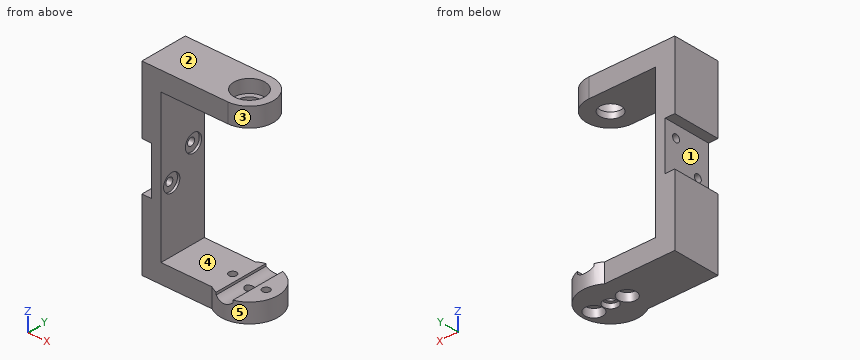
```python
from build123d import *

# Parameters (mm, degrees)
SZKIC25_W                        = 62.15
SZKIC25_H                        = 20
DODANIE_WYCI_GNI_CIE7_DEPTH      = 8
SZKIC14_R                        = 1.75
DODANIE_WYCI_GNI_CIE5_DEPTH      = 8
SZKIC16_R                        = 4.5
DODANIE_WYCI_GNI_CIE6_DEPTH      = 8
SZKIC19_R                        = 6.5
WYTNIJ_WYCI_GNI_CIE8_DEPTH       = 5.5
WYTNIJ_WYCI_GNI_CIE9_REACH       = 94.496
SZKIC20_R                        = 1.6
SZKIC21_R                        = 3.75
WYTNIJ_WYCI_GNI_CIE10_DEPTH      = 3.5
SZKIC22_R                        = 3
WYTNIJ_WYCI_GNI_CIE11_DEPTH      = 2
WYTNIJ_WYCI_GNI_CIE12_REACH      = 68.384
WYTNIJ_WYCI_GNI_CIE12_END_RADIUS = 12
SZKIC26_W                        = 20.2
SZKIC26_H                        = 20
WYTNIJ_WYCI_GNI_CIE13_DEPTH      = 4
WYTNIJ_WYCI_GNI_CIE14_REACH      = 62.057
SZKIC27_R                        = 1.6
SZKIC28_R                        = 3.75
WYTNIJ_WYCI_GNI_CIE15_DEPTH      = 1


with BuildPart() as part:
    # Szkic25 → Dodanie-wyciągnięcie7 (new body)
    with BuildSketch(Plane(origin=(0, 0, 0), x_dir=(0, 0, -1), z_dir=(1, 0, 0))):
        Rectangle(SZKIC25_W, SZKIC25_H)
    extrude(amount=DODANIE_WYCI_GNI_CIE7_DEPTH)

    # Szkic14 → Dodanie-wyciągnięcie5 (add)
    with BuildSketch(Plane(origin=(0, 0, -31.075), x_dir=(-1, 0, 0), z_dir=(0, 0, -1))):
        with BuildLine():
            Line((0, 10), (0, -10))
            Line((0, -10), (-29.366750419, -10))
            ThreePointArc((-29.366750419, -10), (-48, 0), (-29.366750419, 10))
            Line((-29.366750419, 10), (0, 10))
        make_face()
        with Locations((-36, 0)):
            Circle(SZKIC14_R, mode=Mode.SUBTRACT)
    extrude(amount=DODANIE_WYCI_GNI_CIE5_DEPTH)

    # Szkic16 → Dodanie-wyciągnięcie6 (add)
    with BuildSketch(Plane.XY.offset(31.075)):
        with BuildLine():
            Line((0, 10), (0, -10))
            Line((0, -10), (36, -10))
            ThreePointArc((36, -10), (46, 0), (36, 10))
            Line((36, 10), (0, 10))
        make_face()
        with Locations((36, 0)):
            Circle(SZKIC16_R, mode=Mode.SUBTRACT)
    extrude(amount=DODANIE_WYCI_GNI_CIE6_DEPTH)

    # Szkic19 → Wytnij-wyciągnięcie8 (cut)
    with BuildSketch(Plane.XY.offset(39.075)):
        with Locations((36, 0)):
            Circle(SZKIC19_R)
    extrude(amount=-WYTNIJ_WYCI_GNI_CIE8_DEPTH, mode=Mode.SUBTRACT)

    # Szkic20 → Wytnij-wyciągnięcie9 (cut, up to next)
    with BuildSketch(Plane(origin=(0, 0, -39.075), x_dir=(-1, 0, 0), z_dir=(0, 0, -1)), mode=Mode.PRIVATE) as wytnij_wyci_gni_cie9_sk1:
        with Locations(Location((-29, 0, 0), (0, 0, 90))):
            Circle(SZKIC20_R)
    wytnij_wyci_gni_cie9_tool1 = extrude(wytnij_wyci_gni_cie9_sk1.sketch, amount=-WYTNIJ_WYCI_GNI_CIE9_REACH, mode=Mode.PRIVATE) & part.part
    # Szkic20 → Wytnij-wyciągnięcie9 (cut, up to next)
    with BuildSketch(Plane(origin=(0, 0, -39.075), x_dir=(-1, 0, 0), z_dir=(0, 0, -1)), mode=Mode.PRIVATE) as wytnij_wyci_gni_cie9_sk2:
        with Locations(Location((-43, 0, 0), (0, 0, 90))):
            Circle(SZKIC20_R)
    wytnij_wyci_gni_cie9_tool2 = extrude(wytnij_wyci_gni_cie9_sk2.sketch, amount=-WYTNIJ_WYCI_GNI_CIE9_REACH, mode=Mode.PRIVATE) & part.part
    add(wytnij_wyci_gni_cie9_tool1.solids().sort_by_distance((29, 0, -39.075))[0], mode=Mode.SUBTRACT)
    add(wytnij_wyci_gni_cie9_tool2.solids().sort_by_distance((43, 0, -39.075))[0], mode=Mode.SUBTRACT)

    # Szkic21 → Wytnij-wyciągnięcie10 (cut)
    with BuildSketch(Plane(origin=(0, 0, -39.075), x_dir=(-1, 0, 0), z_dir=(0, 0, -1))):
        with Locations(Location((-43, 0, 0), (0, 0, 90))):
            Circle(SZKIC21_R)
        with Locations(Location((-29, 0, 0), (0, 0, 90))):
            Circle(SZKIC21_R)
    extrude(amount=-WYTNIJ_WYCI_GNI_CIE10_DEPTH, mode=Mode.SUBTRACT)

    # Szkic22 → Wytnij-wyciągnięcie11 (cut)
    with BuildSketch(Plane(origin=(0, 0, -39.075), x_dir=(-1, 0, 0), z_dir=(0, 0, -1))):
        with Locations(Location((-36, 0, 0), (0, 0, 90))):
            Circle(SZKIC22_R)
    extrude(amount=-WYTNIJ_WYCI_GNI_CIE11_DEPTH, mode=Mode.SUBTRACT)

    # Wytnij-wyciągnięcie12: up to this cylinder (the profile starts inside it)
    wytnij_wyci_gni_cie12_end = Plane(origin=(36, 0, -32.110303), z_dir=(0, 0, 1)) * Cylinder(WYTNIJ_WYCI_GNI_CIE12_END_RADIUS, 161.768, mode=Mode.PRIVATE)
    # Szkic23 → Wytnij-wyciągnięcie12 (cut, up to the surface)
    with BuildSketch(Plane(origin=(0, 12, 0), x_dir=(1, 0, 0), z_dir=(0, 1, 0)), mode=Mode.PRIVATE) as wytnij_wyci_gni_cie12_sk1:
        with BuildLine():
            Line((32.5, 31.075), (39.5, 31.075))
            Line((39.5, 31.075), (39.5, 32.075))
            ThreePointArc((39.5, 32.075), (36, 33.504285786), (32.5, 32.075))
            Line((32.5, 32.075), (32.5, 31.075))
        make_face()
    wytnij_wyci_gni_cie12_tool1 = extrude(wytnij_wyci_gni_cie12_sk1.sketch, amount=-WYTNIJ_WYCI_GNI_CIE12_REACH, mode=Mode.PRIVATE) & wytnij_wyci_gni_cie12_end
    add(wytnij_wyci_gni_cie12_tool1.solids().sort_by_distance((36, 12, -32.110303))[0], mode=Mode.SUBTRACT)

    # Szkic26 → Wytnij-wyciągnięcie13 (cut)
    with BuildSketch(Plane.ZY):
        with Locations((0.7, 0)):
            Rectangle(SZKIC26_W, SZKIC26_H)
    extrude(amount=-WYTNIJ_WYCI_GNI_CIE13_DEPTH, mode=Mode.SUBTRACT)

    # Szkic27 → Wytnij-wyciągnięcie14 (cut, up to next)
    with BuildSketch(Plane.ZY.offset(-4), mode=Mode.PRIVATE) as wytnij_wyci_gni_cie14_sk1:
        with Locations((5.7, 5)):
            Circle(SZKIC27_R)
    wytnij_wyci_gni_cie14_tool1 = extrude(wytnij_wyci_gni_cie14_sk1.sketch, amount=-WYTNIJ_WYCI_GNI_CIE14_REACH, mode=Mode.PRIVATE) & part.part
    # Szkic27 → Wytnij-wyciągnięcie14 (cut, up to next)
    with BuildSketch(Plane.ZY.offset(-4), mode=Mode.PRIVATE) as wytnij_wyci_gni_cie14_sk2:
        with Locations((-4.250002475, -5.0495025)):
            Circle(SZKIC27_R)
    wytnij_wyci_gni_cie14_tool2 = extrude(wytnij_wyci_gni_cie14_sk2.sketch, amount=-WYTNIJ_WYCI_GNI_CIE14_REACH, mode=Mode.PRIVATE) & part.part
    add(wytnij_wyci_gni_cie14_tool1.solids().sort_by_distance((4, 5, 5.7))[0], mode=Mode.SUBTRACT)
    add(wytnij_wyci_gni_cie14_tool2.solids().sort_by_distance((4, -5.049502, -4.250002))[0], mode=Mode.SUBTRACT)

    # Szkic28 → Wytnij-wyciągnięcie15 (cut)
    with BuildSketch(Plane(origin=(8, 0, 0), x_dir=(0, 0, -1), z_dir=(1, 0, 0))):
        with Locations((-5.7, 5)):
            Circle(SZKIC28_R)
        with Locations((4.250002475, -5.0495025)):
            Circle(SZKIC28_R)
    extrude(amount=-WYTNIJ_WYCI_GNI_CIE15_DEPTH, mode=Mode.SUBTRACT)


solid = part.part
```
Geometry: final body of the model. Coordinates: model frame, mm. Face numbers are marked on the shaded views. A direction names the side the tool comes from. Coordinates: 2 decimals unless noted, no trailing zeros. Loops run counter-clockwise (first coordinate to the right, second up) from the corner with the lowest first, then second, coordinate; pieces in that order, holes last. Notation, with made-up numbers: (45.5, 62.5) -> (95.5, 62.5) arc R23 cw to (95.5, 89.5) -> close; hole circle Ø7 at (76, 7.25). An arc over 180 degrees is marked (long way). Use a Markdown table: item, result. Add a question column.
(1) Pin query (flat end, axial travel): pin 1 Ø2 at (y, z) = (5.5, 7) entering from +X; pin 2 Ø7 at (x, y) = (36, 0) entering from -Z (3 decimals); pin 3 Ø8 at (y, z) = (-5.5, -6) entering from +X; pin 4 Ø1.8 at (x, y) = (36.5, -1.5) entering from -Z (3 decimals). Return the tip coordinate at first contact, or that it passes through.
(2) Mould query, pull axis Z, two halves, no side actions, for the marked faces 1, 2 and 3. Classes: pulls with the +Z half, pulls with the -Z half, needs draft (parallel to the pull), parting line crosses it, or undercut.
(3) Section query B-B, the plane y = 0. State how many separate pieces and enclosed holes the cut face has, plus the area to 3 significant figures.
(4) Access query for the marked faces 4 and 5. Directions: +Z, -Z, +X, -X, +Y, -Y. A direction counts if a zero-diameter tool reaches every point of the face in a straight line with its end or side. Return the directions, or none.
(5) Section query C-C, the plane z = -30. Return loops of the section in (x, y), plus the area to 3 significant figures.
(6) Line query: line 1 along X through (y, z) = (0, -36.45); line 2 along Z through (x, y) = (14, 5) (3 decimals); line 3 along Z through (x, y) = (28.5, 2.75) (3 decimals). Output: solid intervals per line, ascending.
(7) Section query A-A, the plane x = 13.5. Return loops of the section in (y, z) (3 decimals).
Answer:
| question | item | result |
|---|---|---|
| 1 | pin 1 | stops at x = 7 |
| 1 | pin 2 | stops at z = -39.075 |
| 1 | pin 3 | stops at x = 8 |
| 1 | pin 4 | stops at z = -37.075 |
| 2 | face 1 | undercut |
| 2 | face 2 | pulls with the +Z half |
| 2 | face 3 | needs draft |
| 3 | separate pieces | 5 |
| 3 | enclosed holes | 0 |
| 3 | area | 954 mm^2 |
| 4 | face 4 | +X, +Y, -Y |
| 4 | face 5 | +Z, -Z |
| 5 | outline | (0, -10) -> (8, -10) -> (8, 10) -> (0, 10) -> close |
| 5 | area | 160 mm^2 |
| 6 | line 1 | x = 0 to 25.25, 32.75 to 34.25, 37.75 to 39.25, 46.75 to 48 |
| 6 | line 2 | z = -39.075 to -31.075, 31.075 to 39.075 |
| 6 | line 3 | z = -35.575 to -31.075, 31.075 to 39.075 |
| 7 | outline | (-10, -39.075) -> (10, -39.075) -> (10, -31.075) -> (-10, -31.075) -> close; (-10, 31.075) -> (10, 31.075) -> (10, 39.075) -> (-10, 39.075) -> close |
